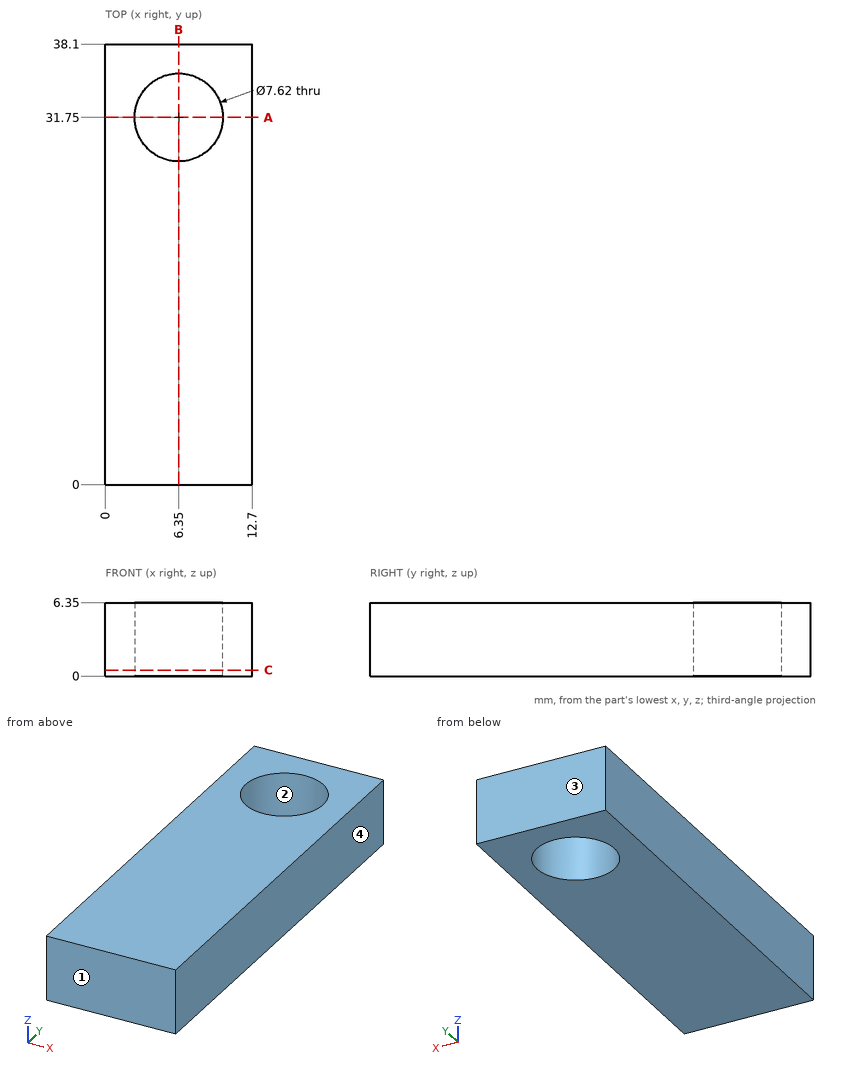
For this review, use the dimensioned drawing (mm, ordinates from the lowest corner) and the shaded views. Coordinates: 2 decimals unless noted, no trailing zeros. Loops run counter-clockwise (first coordinate to the right, second up) from the corner with the lowest first, then second, coordinate; pieces in that order, holes last. Notation, with made-up numbers: (61.25, 83) -> (83.25, 83) arc R17 cw to (83.25, 100) -> close; hole circle Ø5 at (29, 4.25). An arc over 180 degrees is marked (long way). Return JSON: item names as keys, results as strings. Group by question number.
(1) Consider section B-B, the plane x = 6.35. Give the boundary of the cut face in (y, z).
(2) To check wall thickness, follow L1, parallel to Y at x = 6.35, z = 1.75; L2, parallel to X at y = 31.75, z = 2; L3, parallel to X at y = 33.5, z = 1.75. State the ranges of each line that lie inside material, in increasing order.
(3) Consider section C-C, the plane z = 0.5. Give the boundary of the cut face in (x, y), plus the area to 3 significant figures.
(4) Consider section A-A, the plane y = 31.75. Give the boundary of the cut face in (x, z).
(5) Mouldability with a two-part tool opening along Y and no side actions: class the marked faces 1, 2, 3 and 4 as pulls with the +Y half, pulls with the -Y half, needs draft (parallel to the pull), parting line crosses it, or undercut.
Results below:
{
 "1": {"outline": "(0, 0) -> (27.94, 0) -> (27.94, 6.35) -> (0, 6.35) -> close; (35.56, 0) -> (38.1, 0) -> (38.1, 6.35) -> (35.56, 6.35) -> close"},
 "2": {"L1": "y = 0 to 27.94, 35.56 to 38.1", "L2": "x = 0 to 2.54, 10.16 to 12.7", "L3": "x = 0 to 2.97, 9.73 to 12.7"},
 "3": {"outline": "(0, 0) -> (12.7, 0) -> (12.7, 38.1) -> (0, 38.1) -> close; hole circle Ø7.62 at (6.35, 31.75)", "area": "438 mm2"},
 "4": {"outline": "(0, 0) -> (2.54, 0) -> (2.54, 6.35) -> (0, 6.35) -> close; (10.16, 0) -> (12.7, 0) -> (12.7, 6.35) -> (10.16, 6.35) -> close"},
 "5": {"face 1": "pulls with the -Y half", "face 2": "undercut", "face 3": "pulls with the +Y half", "face 4": "needs draft"}
}
